```python
from build123d import *

# Parameters (mm, degrees)
SKIZZE2_W                            = 5
SKIZZE2_H                            = 20
SCHNITT_LINEAR_AUSTRAGEN1_DEPTH      = 49.023431781
SCHNITT_LINEAR_AUSTRAGEN2_DEPTH      = 47.233105022
SCHNITT_LINEAR_AUSTRAGEN2_DEPTH_BACK = 47.233105022
SKIZZE5_R                            = 3


with BuildPart() as part:
    # Skizze1 → Rotation2 (revolve)
    with BuildSketch(Plane.XY, mode=Mode.PRIVATE) as rotation2_sk:
        Polygon((0, -45), (0, 45), (-7.5, 45), (-7.5, 41), (-7, 41), (-7, 40), (-7.5, 40), (-7.5, 37), (-7, 37), (-7, 36), (-7.5, 36), (-7.5, -45), align=None)
    revolve(rotation2_sk.sketch.rotate(Axis((0, -45, 0), (0, 1, 0)), 180), axis=Axis((0, -45, 0), (0, 1, 0)))

    # Skizze2 → Schnitt-Linear austragen1 (cut, through all)
    with BuildSketch(Plane.XY.offset(7.5)):
        with Locations((0, -35)):
            Rectangle(SKIZZE2_W, SKIZZE2_H)
    extrude(amount=-SCHNITT_LINEAR_AUSTRAGEN1_DEPTH, mode=Mode.SUBTRACT)

    # Skizze5 → Schnitt-Linear austragen2 (cut, two sides: drawn at the far end of the back side and taken through both)
    with BuildSketch(Plane(origin=(0, 0, 0), x_dir=(0, 0, -1), z_dir=(1, 0, 0)).offset(-SCHNITT_LINEAR_AUSTRAGEN2_DEPTH_BACK)):
        with Locations(Location((0, -35, 0), (0, 0, 90))):
            Circle(SKIZZE5_R)
    extrude(amount=SCHNITT_LINEAR_AUSTRAGEN2_DEPTH + SCHNITT_LINEAR_AUSTRAGEN2_DEPTH_BACK, mode=Mode.SUBTRACT)


solid = part.part
```
The model under review builds one solid part; all positions refer to its coordinate system, in mm. A direction names the side the tool comes from. Give positions to 0.01 mm unless a question says otherwise; leave off trailing zeros. Loops run counter-clockwise (first coordinate to the right, second up) from the corner with the lowest first, then second, coordinate; pieces in that order, holes last. Notation, with made-up numbers: (40.25, -40) - (98.25, -40) arc R32 ccw to (98.25, -8) - close; hole circle Ø7 at (3, 52). An arc over 180 degrees is marked (long way). Answer as a JSON object with one key per item and string values.
Q1. Add section A-A on z = 0. Count the separate pieces of the cut face and the enclosed holes in it, plus the area to 3 significant figures.
Worked out:
{"separate pieces": "3", "enclosed holes": "0", "area": "1,190 mm^2"}
Q2. Add section C-C on y = -35. State the section outline as (x, z) points.
Worked out:
{"outline": "(-6.87, -3) arc R7.5 ccw to (-2.5, -7.07) - (-2.5, -3) - close; (-6.87, 3) - (-2.5, 3) - (-2.5, 7.07) arc R7.5 ccw to start; (2.5, -7.07) arc R7.5 ccw to (6.87, -3) - (2.5, -3) - close; (2.5, 3) - (6.87, 3) arc R7.5 ccw to (2.5, 7.07) - close"}
Q3. Add section B-B on x = 0. State the section outline as (y, z) points, plus the area to 3 significant figures.
Worked out:
{"outline": "(-25, -7.5) - (36, -7.5) - (36, -7) - (37, -7) - (37, -7.5) - (40, -7.5) - (40, -7) - (41, -7) - (41, -7.5) - (45, -7.5) - (45, 7.5) - (41, 7.5) - (41, 7) - (40, 7) - (40, 7.5) - (37, 7.5) - (37, 7) - (36, 7) - (36, 7.5) - (-25, 7.5) - close", "area": "1,050 mm^2"}
Q4. Mouldability with a two-part tool opening along X and no side actions: class faces 4 (the cylindrical face through (4.032, 42.972, -6.324)), 5 (the flat face through (4, -45, 0)), 6 (the flat face through (0, -25, 0)) as +X half, -X half, draft (parallel to the pull), parting line (faces both ways), or undercut.
Worked out:
{"face 4": "parting line", "face 5": "draft", "face 6": "undercut"}
Q5. Insertion check: pin 1 (8 mm diameter, centred on y = -35, z = 0, fed in from -X); pin 2 (4 mm diameter, centred on y = -32, z = -3.5, fed in from +X); pin 3 (3 mm diameter, centred on x = 3, y = -17, fed in from -Z); pin 4 (3.5 mm diameter, centred on y = -35, z = 0, fed in from +X). Each pin has a flat end and moves straight along its axis. Give the tip position at first contact, or say it passes through.
Worked out:
{"pin 1": "stops at x = -7.5", "pin 2": "stops at x = 7.35", "pin 3": "stops at z = -7.35", "pin 4": "passes through"}
Q6. For faces 1 (the flat face through (2, 36, 7)), 2 (the flat face through (2.5, -35.1, 3.2)), 3 (the cylindrical face through (7.154, -5.067, -2.253)), list the 3-axis set-ups (+Z, -Z, +X, -X, +Y, -Y) from which the entire face can be reached by the end or side of a thin tool; tool diameter is ignored.
Worked out:
{"face 1": "none", "face 2": "+Z, -Z, -Y", "face 3": "+Y, -Y"}
Q7. To check wall thickness, follow line 1 along Y through (x, z) = (-5.6, 0); line 2 along Y through (x, z) = (1.25, 4.25); line 3 along Z through (x, y) = (0.25, -16.5). State the ranges of each line that lie inside material, in increasing order.
Worked out:
{"line 1": "y = -45 to -38, -32 to 45", "line 2": "y = -25 to 45", "line 3": "z = -7.5 to 7.5"}
Q8. Add section D-D on x = 5.5. State the section outline as (y, z) points.
Worked out:
{"outline": "(-45, -5.1) - (36, -5.1) - (36, -4.33) - (37, -4.33) - (37, -5.1) - (40, -5.1) - (40, -4.33) - (41, -4.33) - (41, -5.1) - (45, -5.1) - (45, 5.1) - (41, 5.1) - (41, 4.33) - (40, 4.33) - (40, 5.1) - (37, 5.1) - (37, 4.33) - (36, 4.33) - (36, 5.1) - (-45, 5.1) - close; hole circle Ø6 at (-35, 0)"}
